Model file for the job. Use its own axes, mm. A direction names the side the tool comes from. Coordinates: 2 decimals unless noted, no trailing zeros. Write each loop counter-clockwise with the first axis right and the second up, starting at its lowest first coordinate (ties: lowest second). Pieces come first, ordered by that corner, then holes. Notation, with made-up numbers: (25.5, -16.5) - (59.5, -16.5) arc R27 ccw to (59.5, 20.5) - close; hole circle Ø2 at (-11, -14). An arc over 180 degrees is marked (long way). Put each result on its own line as item: value. Start each with the question number.
1. Saw through at B-B, the plane x = 0. Write the cut outline in (y, z).
2. Pull direction Y, two halves, no side cores. Call faces 6 (the face through (8.196, 13.711, -7.266)), 7 (the face through (48, -8, 24)), 8 (the face through (17.414, 20.774, 10.208)): released by +Y, released by -Y, zero draft, split by the parting line, or undercut.
3. Drill centre lines: L1, parallel to Y at x = 30, z = 20; L2, parallel to Y at x = 0, z = 4; L3, parallel to X at y = 20, z = 22. Where is each one in solid material? Low to high. Write a range as from..to.
4. Drop flat-ended pins along their axis: P1, Ø0.6, axis at y = 26.5, z = 10.5, coming from the +X side; P2, Ø3, axis at y = 23, z = 7.5, coming from the +X side; P3, Ø4.5, axis at x = 35.5, z = 23.5, coming from the +Y side. Give the stop position or say it passes through.
5. Saw through at D-D, the plane z = -15. Write the cut outline in (x, y).
6. Saw through at A-A, the plane y = -23.5. Write the cut outline in (x, z), plus the area to 3 significant figures.
7. Saw through at C-C, the plane y = -8. Write the cut outline in (x, z), plus the area to 3 significant figures.
8. Which spindle directions (+Z, -Z, +X, -X, +Y, -Y) get a long thin tool onto all of the face, cutting with end or side? Do faces 1 (the face through (15.5, 22, 8)), 2 (the face through (14.9, 29.43, 18.9)), 3 (the face through (28.07, 19.203, 24.859)), 4 (the face through (-9, 21.75, 0)), 5 (the face through (35.44, 20.77, 9.65)). Say none if no direction does.
```python
from build123d import *

# Parameters (mm, degrees)
RESSALTO_EXTRUS_O2_DEPTH   = 26
ESBO_O4_W                  = 38
ESBO_O4_H                  = 42
CORTE_EXTRUS_O1_DEPTH      = 45.452221542
ESBO_O5_W                  = 14
ESBO_O5_H                  = 60
RESSALTO_EXTRUS_O3_DEPTH   = 47
ESBO_O8_R                  = 1.6
ESBO_O8_R_2                = 12
CORTE_EXTRUS_O3_DEPTH      = 83.782848465
ESBO_O6_R                  = 4.1
CORTE_EXTRUS_O4_DEPTH      = 15
CORTE_EXTRUS_O5_REACH      = 79.878
CORTE_EXTRUS_O5_END_RADIUS = 12
ESBO_O10_W                 = 10
ESBO_O10_H                 = 15
ESBO_O12_W                 = 25
ESBO_O12_H                 = 12
RESSALTO_EXTRUS_O4_DEPTH   = 6
CORTE_EXTRUS_O6_DEPTH      = 75.786362393
CORTE_EXTRUS_O6_DEPTH_BACK = 75.786362393
ESBO_O11_W                 = 25
ESBO_O11_H                 = 3
ESBO_O13_W                 = 10
ESBO_O13_H                 = 6
CORTE_EXTRUS_O7_DEPTH      = 75.786362393
FILETE5_R                  = 4
FILETE6_R                  = 6
FILETE8_R                  = 2
FILETE9_R                  = 2
ESBO_O14_R                 = 1.6
CORTE_EXTRUS_O8_DEPTH      = 8
ESBO_O15_W                 = 5.8
ESBO_O15_H                 = 2.5
CORTE_EXTRUS_O9_DEPTH      = 7
CORTE_EXTRUS_O10_DEPTH     = 5
PADR_O_LINEAR1_COUNT       = 10
PADR_O_LINEAR1_PITCH       = 2
FILETE10_R                 = 0.3
CHANFRO1_SIZE              = 25


with BuildPart() as part:
    # Esboço1 → Ressalto-extrusão2 (new, symmetric)
    with BuildSketch(Plane.XY):
        with BuildLine():
            Line((10, 30), (-10, 30))
            Line((-10, 30), (-10, 21.75))
            Line((-10, 21.75), (-7.462405778, 21.75))
            ThreePointArc((-7.462405778, 21.75), (0.375470813, 28.490595548), (7.5, 21))
            ThreePointArc((7.5, 21), (0.375470813, 13.509404452), (-7.462405778, 20.25))
            Line((-7.462405778, 20.25), (-10, 20.25))
            Line((-10, 20.25), (-10, -30))
            Line((-10, -30), (10, -30))
            Line((10, -30), (10, 30))
        make_face()
    extrude(amount=RESSALTO_EXTRUS_O2_DEPTH, both=True)

    # Esboço4 → Corte-extrusão1 (cut, through all)
    with BuildSketch(Plane(origin=(10, 0, 0), x_dir=(0, 0, -1), z_dir=(1, 0, 0))):
        with Locations((7, -9)):
            Rectangle(ESBO_O4_W, ESBO_O4_H)
    extrude(amount=-CORTE_EXTRUS_O1_DEPTH, mode=Mode.SUBTRACT)

    # Esboço5 → Ressalto-extrusão3 (add)
    with BuildSketch(Plane(origin=(10, 0, 0), x_dir=(0, 0, -1), z_dir=(1, 0, 0))):
        with Locations((-19, 0)):
            Rectangle(ESBO_O5_W, ESBO_O5_H)
    extrude(amount=RESSALTO_EXTRUS_O3_DEPTH)

    # Esboço8 → Corte-extrusão3 (cut, through all)
    with BuildSketch(Plane.XY.offset(26)):
        with Locations((45.5, 7.5)):
            Circle(ESBO_O8_R)
        with Locations((14.5, -23.5)):
            Circle(ESBO_O8_R)
        with Locations((30, -8)):
            Circle(ESBO_O8_R_2)
        with Locations((14.5, 7.5)):
            Circle(ESBO_O8_R)
    extrude(amount=-CORTE_EXTRUS_O3_DEPTH, mode=Mode.SUBTRACT)

    # Esboço6 → Corte-extrusão4 (cut)
    with BuildSketch(Plane(origin=(57, 0, 0), x_dir=(0, 0, -1), z_dir=(1, 0, 0))):
        with Locations(Location((-19, 23.5, 0), (0, 0, 90))):
            Circle(ESBO_O6_R)
        with Locations(Location((-19, -23.5, 0), (0, 0, 270))):
            Circle(ESBO_O6_R)
    extrude(amount=-CORTE_EXTRUS_O4_DEPTH, mode=Mode.SUBTRACT)

    # Corte-extrusão5: up to this cylinder (the profile starts outside it)
    corte_extrus_o5_end = Plane(origin=(30, -8, 19), z_dir=(0, 0, 1)) * Cylinder(CORTE_EXTRUS_O5_END_RADIUS, 184.756, mode=Mode.PRIVATE)
    # Esboço10 → Corte-extrusão5 (cut, up to the surface)
    with BuildSketch(Plane(origin=(57, 0, 0), x_dir=(0, 0, -1), z_dir=(1, 0, 0)), mode=Mode.PRIVATE) as corte_extrus_o5_sk1:
        with Locations((-19, -8)):
            Rectangle(ESBO_O10_W, ESBO_O10_H)
    corte_extrus_o5_tool1 = extrude(corte_extrus_o5_sk1.sketch, amount=-CORTE_EXTRUS_O5_REACH, mode=Mode.PRIVATE) - corte_extrus_o5_end
    add(corte_extrus_o5_tool1.solids().sort_by_distance((57, -8, 19))[0], mode=Mode.SUBTRACT)

    # Esboço12 → Ressalto-extrusão4 (add)
    with BuildSketch(Plane(origin=(0, 0, 12), x_dir=(-1, 0, 0), z_dir=(0, 0, -1))):
        with Locations((-28, 24)):
            Rectangle(ESBO_O12_W, ESBO_O12_H)
    extrude(amount=RESSALTO_EXTRUS_O4_DEPTH)

    # Esboço11 → Corte-extrusão6 (cut, two sides: drawn at the far end of the back side and taken through both)
    with BuildSketch(Plane(origin=(0, 0, 12), x_dir=(-1, 0, 0), z_dir=(0, 0, -1)).offset(-CORTE_EXTRUS_O6_DEPTH_BACK)):
        with Locations((-28, 28.5)):
            Rectangle(ESBO_O11_W, ESBO_O11_H)
    extrude(amount=CORTE_EXTRUS_O6_DEPTH + CORTE_EXTRUS_O6_DEPTH_BACK, mode=Mode.SUBTRACT)

    # Esboço13 → Corte-extrusão7 (cut, through all)
    with BuildSketch(Plane(origin=(0, 0, 12), x_dir=(-1, 0, 0), z_dir=(0, 0, -1))):
        with Locations((-28, 15)):
            Rectangle(ESBO_O13_W, ESBO_O13_H)
    extrude(amount=-CORTE_EXTRUS_O7_DEPTH, mode=Mode.SUBTRACT)

    # Filete5
    filete5_edges = [part.edges().sort_by_distance(p)[0] for p in [
        (28, 18, 6),
        (28, 12, 26),
        (28, 18, 26),
        (28, 12, 12),
    ]]
    fillet(filete5_edges, radius=FILETE5_R)

    # Filete6
    filete6_edges = [part.edges().sort_by_distance(p)[0] for p in [
        (-10, 30, 0),
        (-10, 12, -7),
        (10, 12, -7),
        (10, 30, -7),
    ]]
    fillet(filete6_edges, radius=FILETE6_R)

    # Filete8
    filete8_edges = [part.edges().sort_by_distance(p)[0] for p in [
        (40.5, 22.5, 12),
        (15.5, 22.5, 12),
    ]]
    fillet(filete8_edges, radius=FILETE8_R)

    # Filete9
    filete9_edges = [part.edges().sort_by_distance(p)[0] for p in [
        (15.5, 30, 19),
        (40.5, 30, 19),
    ]]
    fillet(filete9_edges, radius=FILETE9_R)

    # Esboço14 → Corte-extrusão8 (cut)
    with BuildSketch(Plane(origin=(0, 27, 0), x_dir=(1, 0, 0), z_dir=(0, 1, 0))):
        with Locations(Location((19, -22, 0), (0, 0, 270))):
            Circle(ESBO_O14_R)
        with Locations(Location((37, -22, 0), (0, 0, 90))):
            Circle(ESBO_O14_R)
        with Locations(Location((37, -10, 0), (0, 0, 270))):
            Circle(ESBO_O14_R)
        with Locations(Location((19, -10, 0), (0, 0, 90))):
            Circle(ESBO_O14_R)
    extrude(amount=-CORTE_EXTRUS_O8_DEPTH, mode=Mode.SUBTRACT)

    # Esboço15 → Corte-extrusão9 (cut)
    with BuildSketch(Plane.XY.offset(26)):
        with Locations((19, 23.75)):
            Rectangle(ESBO_O15_W, ESBO_O15_H)
        with Locations((37, 23.75)):
            Rectangle(ESBO_O15_W, ESBO_O15_H)
    corte_extrus_o9 = extrude(amount=-CORTE_EXTRUS_O9_DEPTH, mode=Mode.SUBTRACT)

    # Espelhar1: Corte-extrusão9 across plane
    add(corte_extrus_o9.mirror(Plane.XY.offset(16)), mode=Mode.SUBTRACT)

    # Esboço16 → Corte-extrusão10 (cut, symmetric)
    with BuildSketch(Plane(origin=(28, 0, 0), x_dir=(0, 0, -1), z_dir=(1, 0, 0))):
        with BuildLine():
            Line((-7.7, 27), (-6.3, 27))
            ThreePointArc((-6.3, 27), (-7, 26.3), (-7.7, 27))
        make_face()
    corte_extrus_o10 = extrude(amount=CORTE_EXTRUS_O10_DEPTH, both=True, mode=Mode.SUBTRACT)

    # Padrão linear1: Corte-extrusão10 ×10
    with Locations(*[(0, 0, i * PADR_O_LINEAR1_PITCH) for i in range(1, PADR_O_LINEAR1_COUNT)]):
        add(corte_extrus_o10, mode=Mode.SUBTRACT)

    # Filete10
    filete10_edges = [part.edges().sort_by_distance(p)[0] for p in [
        (28, 27, 7.7),
        (28, 27, 6.3),
        (28, 27, 9.7),
        (28, 27, 8.3),
        (28, 27, 11.7),
        (28, 27, 10.3),
        (28, 27, 13.7),
        (28, 27, 12.3),
        (28, 27, 15.7),
        (28, 27, 14.3),
        (28, 27, 17.7),
        (28, 27, 16.3),
        (28, 27, 19.7),
        (28, 27, 18.3),
        (28, 27, 21.7),
        (28, 27, 20.3),
        (28, 27, 23.7),
        (28, 27, 22.3),
        (28, 27, 24.3),
    ]]
    fillet(filete10_edges, radius=FILETE10_R)

    # Chanfro1
    chanfro1_edges = [part.edges().sort_by_distance(p)[0] for p in [
        (-10, -30, 19),
    ]]
    chamfer(chanfro1_edges, length=CHANFRO1_SIZE)


solid = part.part
```
Final values:
1. outline: (-15, 12) - (12, 12) - (12, -26) - (13.5, -26) - (13.5, 26) - (-15, 26) - close; (28.5, -26) - (30, -26) - (30, 26) - (28.5, 26) - close
2. face 6: released by -Y
2. face 7: undercut
2. face 8: zero draft
3. L1: y = -30..-20, 4..12, 18..27
3. L2: y = 12..13.5, 28.5..30
3. L3: x = -10..-7.43, 7.43..17.4, 20.6..35.4, 38.6..57
4. P1: stops at x = 40.67
4. P2: stops at x = 40.5
4. P3: stops at y = 27
5. outline: (-10, 18) arc R6 ccw to (-4, 12) - (4, 12) arc R6 ccw to (10, 18) - (10, 24) arc R6 ccw to (4, 30) - (-4, 30) arc R6 ccw to (-10, 24) - (-10, 21.75) - (-7.46, 21.75) arc R7.5 cw (long way) to (-7.46, 20.25) - (-10, 20.25) - close
6. outline: (8.5, 12) - (12.9, 12) - (12.9, 26) - (8.5, 26) - close; (16.1, 12) - (57, 12) - (57, 14.9) - (42, 14.9) - (42, 23.1) - (57, 23.1) - (57, 26) - (16.1, 26) - close
6. area: 511 mm²
7. outline: (-7, 12) - (18, 12) - (18, 26) - (-7, 26) - close; (42, 12) - (57, 12) - (57, 14) - (42, 14) - close; (42, 24) - (57, 24) - (57, 26) - (42, 26) - close
7. area: 410 mm²
8. face 1: -Z, +Y, -Y
8. face 2: +Z, -Z, +Y
8. face 3: +Z
8. face 4: +Z, -Z, -X
8. face 5: +Y
